from build123d import *

# Parameters (mm, degrees)
CYLINDER009_R          = 11
CYLINDER009_DEPTH      = 61
BOX020_W               = 32
BOX020_H               = 32
BOX020_DEPTH           = 8
BOX020_PLACEMENT_ANGLE = 10
CYLINDER008_R          = 14
CYLINDER008_DEPTH      = 61
CUT014_PLACEMENT_ANGLE = 8


with BuildPart() as obj1:
    # Cylinder009 → Cylinder009 (new body)
    with BuildSketch(Plane(origin=(15, -20, -39), x_dir=(1, 0, 0), z_dir=(0, 0, 1))):
        Circle(CYLINDER009_R)
    extrude(amount=CYLINDER009_DEPTH)


with BuildPart() as fusion010:
    # Box020 → Box020 (new body)
    with BuildSketch(Plane.XY):
        with Locations((16, 16)):
            Rectangle(BOX020_W, BOX020_H)
    extrude(amount=BOX020_DEPTH)


with BuildPart() as fusion010_1:
    # Box020 placement: moved
    add(fusion010.part.moved(Location((-2, -36, 25))).rotate(Axis((-2, -36, 25), (-1, 0, 0)), BOX020_PLACEMENT_ANGLE))

    # Fusion010: union obj1
    add(obj1.part)


with BuildPart() as tube:
    # Cylinder008 → Cylinder008 (new body)
    with BuildSketch(Plane(origin=(15, -20, -39), x_dir=(1, 0, 0), z_dir=(0, 0, 1))):
        Circle(CYLINDER008_R)
    extrude(amount=CYLINDER008_DEPTH)

    # Cut014: cut Fusion010
    add(fusion010_1.part, mode=Mode.SUBTRACT)


with BuildPart() as tube_1:
    # Cut014 placement: moved
    add(tube.part.moved(Location((0, 5, 3))).rotate(Axis((0, 5, 3), (1, 0, 0)), CUT014_PLACEMENT_ANGLE))


solid = tube_1.part
CAD build for the part. Positions are in the model's coordinates, mm. Round coordinates to 2 decimals unless told otherwise and drop trailing zeros. Write each loop counter-clockwise with the first axis right and the second up, starting at its lowest first coordinate (ties: lowest second). Pieces come first, ordered by that corner, then holes. Notation, with made-up numbers: M -37.5,71 L -33.5,71 A13 ccw -33.5,87 Z; hole C -34.75,80 d1. An arc over 180 degrees is marked long. Put each result on its own line as item: value. Start each with the question number.
1) Drill centre lines: probe 1 along Y at (x, z) = (6.25, 19.5); probe 2 along X at (y, z) = (-8.5, -20); probe 3 along Y at (x, z) = (18.25, 3). Where is each one in solid material? Low to high. Write a range as [from, to].
2) Pin check, flat tips, straight feed: pin 1 Ø3 at (y, z) = (0, -5.5) entering from -X; pin 2 Ø3 at (x, z) = (15.5, -16.5) entering from +Y; pin 3 Ø3 at (x, y) = (18, -20.5) entering from -Z. Stop position of each tip, or through.
3) Saw through at A-A, the plane x = 23.5. Write the cut outline in (y, z).
4) Pull direction Z, two halves, no side cores. Call faces 1 (the flat face through (21.2, -18.6, -39.7)), 2 (the cylindrical face through (27.932, -18.873, -9.37)), 3 (the cylindrical face through (20.914, -4.378, -7.333)): pulls with the +Z half, pulls with the -Z half, needs draft (parallel to the pull), parting line crosses it, or undercut.
5) Saw through at B-B, the plane x = 17.5. Write the cut outline in (y, z).
Resolved:
1. probe 1: [-28.55, -24.25], [-10.78, -6.48]
1. probe 2: [1.43, 4.55], [25.45, 28.57]
1. probe 3: [-28.95, -25.81], [-4.58, -1.45]
2. pin 1: x = 8.44
2. pin 2: y = 1.89
2. pin 3: z = -40.18
3. outline: M -28.88,20.45 L -20.39,-39.95 L -16.29,-39.38 L -24.78,21.03 Z; M -10.81,21.93 L -2.46,-37.43 L 1.64,-36.86 L -6.6,21.79 Z
4. face 1: pulls with the -Z half
4. face 2: parting line crosses it
4. face 3: undercut
5. outline: M -31.51,20.09 L -23.02,-40.32 L -19.99,-39.89 L -28.48,20.51 Z; M -7.02,21.8 L 1.23,-36.91 L 4.26,-36.49 L -3.91,21.69 Z
